Geometry: final body of the model. Coordinates: model frame, mm. A direction names the side the tool comes from. Round coordinates to 2 decimals unless told otherwise and drop trailing zeros. Loops run counter-clockwise (first coordinate to the right, second up) from the corner with the lowest first, then second, coordinate; pieces in that order, holes last. Notation, with made-up numbers: M 70,18.5 L 114,18.5 A21 ccw 114,39.5 Z; hole C 72,3 d7. An arc over 180 degrees is marked long. Answer as a JSON object with one key per item and string values.
from build123d import *

# Parameters (mm, degrees)
SCHIZZO1_R                   = 6.25
ESTRUSIONE_ESTRUSIONE1_DEPTH = 10
RACCORDO1_R                  = 11
SCHIZZO2_R                   = 1.863588926
TAGLIO_ESTRUSIONE1_DEPTH     = 10


with BuildPart() as part:
    # Schizzo1 → Estrusione-Estrusione1 (new body)
    with BuildSketch(Plane(origin=(0, 0, 0), x_dir=(1, 0, 0), z_dir=(0, 1, 0))):
        Polygon((0, 0), (0, -37.9), (0, -65.7), (42.8, -22.9), (42.8, 0), align=None)
        with Locations(Location((11, -37.9, 0), (0, 0, 270))):
            Circle(SCHIZZO1_R, mode=Mode.SUBTRACT)
        with Locations(Location((28.6, -19, 0), (0, 0, 270))):
            Circle(SCHIZZO1_R, mode=Mode.SUBTRACT)
    extrude(amount=ESTRUSIONE_ESTRUSIONE1_DEPTH)

    # Raccordo1
    raccordo1_edges = [part.edges().sort_by_distance(p)[0] for p in [
        (0, 5, 65.7),
    ]]
    fillet(raccordo1_edges, radius=RACCORDO1_R)

    # Schizzo2 → Taglio-Estrusione1 (cut)
    with BuildSketch(Plane.ZY):
        with Locations((3, 5)):
            Circle(SCHIZZO2_R)
        with Locations((9, 5)):
            Circle(SCHIZZO2_R)
    extrude(amount=-TAGLIO_ESTRUSIONE1_DEPTH, mode=Mode.SUBTRACT)


solid = part.part
1) Ray query, line 1 (Y direction, x = 6.25, z = 9); line 2 (X direction, y = 3, z = 19); line 3 (Z direction, x = 3.5, y = 5.25). Return the intervals inside material, ascending.
Results:
{"line 1": "0 to 3.14, 6.86 to 10", "line 2": "0 to 22.35, 34.85 to 42.8", "line 3": "0 to 1.15, 4.85 to 7.15, 10.85 to 47.19"}
2) Pull-direction query (Z, two-part tool) for faces 3 (the flat face through (21, 10, 19)), 4 (the flat face through (10, 5, 9)), 5 (the flat face through (22, 5, 0)); classes: +Z half, -Z half, draft (parallel to the pull), parting line (faces both ways), or undercut.
Results:
{"face 3": "draft", "face 4": "undercut", "face 5": "-Z half"}
3) Reachability of faces 1 (the flat face through (10, 5, 3)), 2 (the cylindrical face through (24.8, 4.93, 14.04)) from +Z, -Z, +X, -X, +Y, -Y: full face, straight path, thin tool, end or side. Return the list, or none.
Results:
{"face 1": "-X", "face 2": "+Y, -Y"}
4) Section query D-D (y = 5). Return the cut outline in (x, z), and give its area (3 significant figures).
Results:
{"outline": "M 0,0 L 42.8,0 L 42.8,22.9 L 18.78,46.92 A11 ccw 0,39.14 L 0,10.86 L 10,10.86 L 10,7.14 L 0,7.14 L 0,4.86 L 10,4.86 L 10,1.14 L 0,1.14 Z; hole C 11,37.9 d12.5; hole C 28.6,19 d12.5", "area": "1,430 mm2"}
5) Section query A-A (x = 11). Return the cut outline in (y, z), and give its area (3 significant figures).
Results:
{"outline": "M 0,0 L 10,0 L 10,31.65 L 0,31.65 Z; M 0,44.15 L 10,44.15 L 10,50.14 L 0,50.14 Z", "area": "376 mm2"}
6) Section query C-C (y = 1.5). Return the cut outline in (x, z).
Results:
{"outline": "M 0,0 L 42.8,0 L 42.8,22.9 L 18.78,46.92 A11 ccw 0,39.14 Z; hole C 11,37.9 d12.5; hole C 28.6,19 d12.5"}
7) Section query B-B (z = 19). Return the cut outline in (x, y).
Results:
{"outline": "M 0,0 L 22.35,0 L 22.35,10 L 0,10 Z; M 34.85,0 L 42.8,0 L 42.8,10 L 34.85,10 Z"}
8) Pin query (flat end, axial travel): P1, Ø4, axis at x = 16, y = 6, coming from the +Z side; P2, Ø1.9, axis at y = 5, z = 3, coming from the -X side. Return the tip coordinate at first contact, or that it passes through.
Results:
{"P1": "z = 49.73", "P2": "x = 10"}
